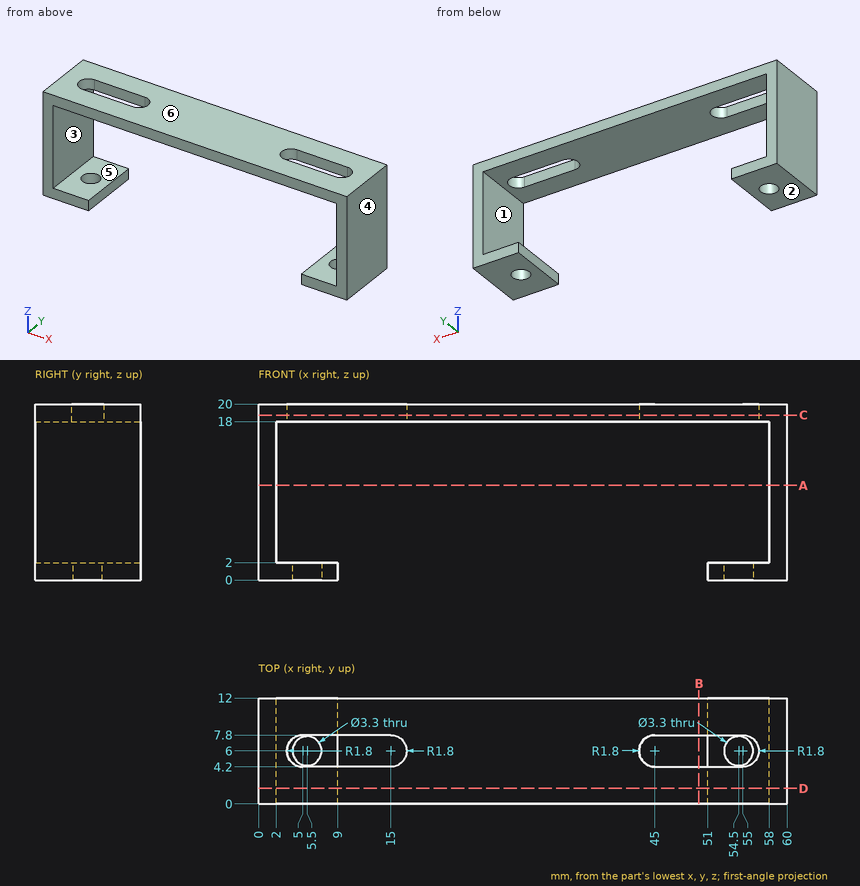
Design review of the part shown in the three views and the two pictorial views. Dimensions are in mm from the part's minimum x, y and z. A direction names the side the tool comes from. Round coordinates to 2 decimals unless told otherwise and drop trailing zeros. Write each loop counter-clockwise with the first axis right and the second up, starting at its lowest first coordinate (ties: lowest second). Pieces come first, ordered by that corner, then holes. Notation, with made-up numbers: M -32,51 L -22,51 A15 cw -22,72 Z; hole C 42.5,4 d9. An arc over 180 degrees is marked long. Use a Markdown table: item, result. Add a question column.
Q1. Machinability: for the marked faces 5 and 6, which of the approach directions +Z, -Z, +X, -X, +Y, -Y give a long, thin tool a straight path to every point of the face, cutting with its end or side? Answer none if there is none.
Q2. We need section B-B, the plane x = 50. State the section outline as (y, z) points, plus the area to 3 significant figures.
Q3. We need section A-A, the plane z = 10.75. State the section outline as (x, y) points, plus the area to 3 significant figures.
Q4. We need section C-C, the plane z = 18.75. State the section outline as (x, y) points, plus the area to 3 significant figures.
Q5. To check wall thickness, follow line 1 (Y direction, x = 54.5, z = 1.6); line 2 (X direction, y = 6.25, z = 12.75); line 3 (Z direction, x = 57, y = 2.75). State the ranges of each line that lie inside material, in increasing order.
Q6. We need section D-D, the plane y = 1.75. State the section outline as (x, z) points.
Q7. The part is to be moulded in two halves that separate along Z. For the marked faces 1, 2, 3 and 4, say which applies: pulls with the +Z half, pulls with the -Z half, needs draft (parallel to the pull), parting line crosses it, or undercut.
Q8. Insertion check: pin 1 (4 mm diameter, centred on x = 13, y = 4, fed in from -Z); pin 2 (3.5 mm diameter, centred on x = 54.5, y = 6, fed in from +Z). Each pin has a flat end and moves straight along its axis. Give the tip position at first contact, or say it passes through.
Findings below:
| question | item | result |
|---|---|---|
| 1 | face 5 | +Y, -Y |
| 1 | face 6 | +Z, +X, -X, +Y, -Y |
| 2 | outline | M 0,18 L 4.2,18 L 4.2,20 L 0,20 Z; M 7.8,18 L 12,18 L 12,20 L 7.8,20 Z |
| 2 | area | 16.8 mm² |
| 3 | outline | M 0,0 L 2,0 L 2,12 L 0,12 Z; M 58,0 L 60,0 L 60,12 L 58,12 Z |
| 3 | area | 48.0 mm² |
| 4 | outline | M 0,0 L 60,0 L 60,12 L 0,12 Z; hole M 5,4.2 L 15,4.2 A1.8 ccw 15,7.8 L 5,7.8 A1.8 ccw Z; hole M 45,4.2 L 55,4.2 A1.8 ccw 55,7.8 L 45,7.8 A1.8 ccw Z |
| 4 | area | 628 mm² |
| 5 | line 1 | y = 0 to 4.35, 7.65 to 12 |
| 5 | line 2 | x = 0 to 2, 58 to 60 |
| 5 | line 3 | z = 0 to 2, 18 to 20 |
| 6 | outline | M 0,0 L 9,0 L 9,2 L 2,2 L 2,18 L 58,18 L 58,2 L 51,2 L 51,0 L 60,0 L 60,20 L 0,20 Z |
| 7 | face 1 | undercut |
| 7 | face 2 | pulls with the -Z half |
| 7 | face 3 | undercut |
| 7 | face 4 | needs draft |
| 8 | pin 1 | stops at z = 18 |
| 8 | pin 2 | stops at z = 2 |
